Autodesk Fusion 360 part; units mm, degrees
sketch "Sketch1" plane through (0, 0, 0) normal (0, 0, 1) x (1, 0, 0)
  circle A0 centre (0, 0) radius 15
  dimension "d1" = 30
extrude "Extrude1" add sketch "Sketch1" along normal blind 6
sketch "Sketch2" plane through (0, 0, 6) normal (0, 0, 1) x (-1, 0, 0)
  circle A0 centre (0, 0) radius 15
  circle A1 centre (-2, -7) radius 12.5
  circle A2 centre (-11, -14) radius 7.5
  dimension "d4" = 25
  dimension "d5" = 15
  dimension "d6" = 7
  dimension "d7" = 2
  dimension "d8" = 14
  dimension "d9" = 11
extrude "Extrude2" add sketch "Sketch2" against normal blind 6 contours A0 A1 A2 picked at (-2.4117, -16.9728)
pattern_circular "C-Pattern1" count 3 over 360 about axis through (0, 0, 6) along (0, 0, 1) of "Extrude2"
sketch "Sketch3" plane through (0, 0, 6) normal (0, 0, 1) x (-1, 0, 0)
  arc A0 (9.6768, -11.4612) -> (14.3884, 4.2397) centre (0, 0) ccw
  arc A1 (19.1866, 4.8092) -> (14.3884, 4.2397) centre (17.6244, -2.5263) ccw
  arc A2 (19.1866, 4.8092) -> (5.0873, 14.111) centre (7.0622, 1.7679) ccw
  arc A3 (5.0873, 14.111) -> (-10.8659, 10.3408) centre (0, 0) ccw
  arc A4 (-13.7582, 14.2114) -> (-10.8659, 10.3408) centre (-6.6244, 16.5263) ccw
  arc A5 (-13.7582, 14.2114) -> (-14.7641, -2.6497) centre (-5.0622, 5.2321) ccw
  arc A6 (-14.7641, -2.6497) -> (-3.5225, -14.5805) centre (0, 0) ccw
  arc A7 (-5.4284, -19.0207) -> (-3.5225, -14.5805) centre (-11, -14) ccw
  arc A8 (-5.4284, -19.0207) -> (9.6768, -11.4612) centre (-2, -7) ccw
  circle A9 centre (0, 0) radius 12
  dimension "d14" = 24
extrude "Extrude3" cut sketch "Sketch3" against normal blind 2 draft -45 contours A9
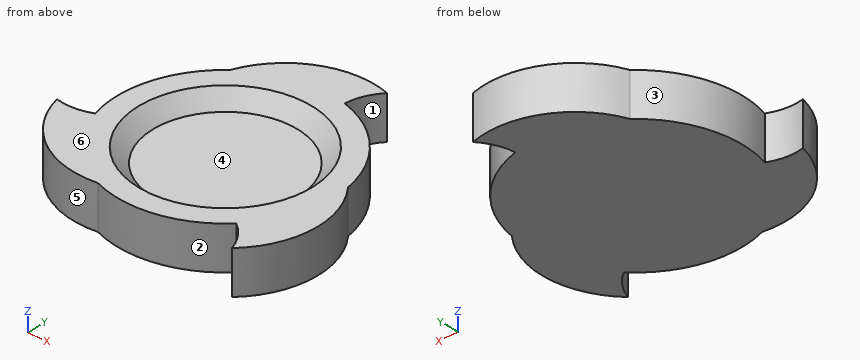
For this review, take the finished solid that the model builds, in its own axes (mm). Face numbers are marked on the shaded views. A direction names the side the tool comes from. Round coordinates to 2 decimals unless told otherwise and drop trailing zeros. Order: outer loops, then holes, each group sorted by start corner. A loop starts at its lowest first (then second) coordinate and runs counter-clockwise, first axis right, second up. Notation, with made-up numbers: (85.5, -38.5) -> (102.5, -38.5) arc R24 cw to (102.5, -19.5) -> close; hole circle Ø10 at (9, 79). An arc over 180 degrees is marked (long way). Put each result on its own line as item: value.
Q1. Add section B-B on x = 0. Write out the cut boundary in (y, z).
Check result:
outline: (-15, 0) -> (19.34, 0) -> (19.34, 6) -> (12, 6) -> (10, 4) -> (-10, 4) -> (-12, 6) -> (-15, 6) -> close
Q2. Add section C-C on y = 0. Write out the cut boundary in (x, z), plus the area to 3 significant figures.
Check result:
outline: (-15, 0) -> (16.41, 0) -> (16.41, 6) -> (12, 6) -> (10, 4) -> (-10, 4) -> (-12, 6) -> (-15, 6) -> close
area: 144 mm2
Q3. Add section D-D on x = -13.5. Write out the cut boundary in (y, z), plus the area to 3 significant figures.
Check result:
outline: (-12.48, 0) -> (6.54, 0) -> (6.54, 6) -> (-12.48, 6) -> close
area: 114 mm2
Q4. Insertion check: pin 1 Ø8 at (x, y) = (3, 8.5) entering from +Z; pin 2 Ø3 at (y, z) = (12.5, 5.5) entering from -X; pin 3 Ø2 at (x, z) = (-9.5, 4) entering from +Y; pin 4 Ø1.5 at (x, y) = (2, 4) entering from +Z. Each pin has a flat end and moves straight along its axis. Give the tip position at first contact, or say it passes through.
Check result:
pin 1: z = 6
pin 2: x = -10.2
pin 3: y = 13.78
pin 4: z = 4
Q5. For probe 1 along Z at (x, y) = (2.5, -3); probe 2 along Y at (x, z) = (-1, 5.25); probe 3 along X at (y, z) = (-13, 2.65), list the stretches that pass through material, from the lowest coordinate up. Write a range as [from, to].
Check result:
probe 1: [0, 4]
probe 2: [-14.97, -11.21], [11.21, 19.13]
probe 3: [-12.55, 7.48], [13.24, 14.86]
Q6. Mouldability with a two-part tool opening along Y and no side actions: class the marked faces 3, 4, 5 and 6 as pulls with the +Y half, pulls with the -Y half, needs draft (parallel to the pull), parting line crosses it, or undercut.
Check result:
face 3: undercut
face 4: undercut
face 5: pulls with the -Y half
face 6: needs draft
Q7. Add section A-A on z = 4.5. Write out the cut boundary in (x, y), plus the area to 3 significant figures.
Check result:
outline: (-19.19, -4.81) arc R12.5 ccw to (-5.09, -14.11) arc R15 ccw to (10.87, -10.34) arc R7.5 cw to (13.76, -14.21) arc R12.5 ccw to (14.76, 2.65) arc R15 ccw to (3.52, 14.58) arc R7.5 cw to (5.43, 19.02) arc R12.5 ccw to (-9.68, 11.46) arc R15 ccw to (-14.39, -4.24) arc R7.5 cw to start; hole circle Ø21 at (0, 0)
area: 505 mm2
Q8. Machinability: for the marked faces 1 and 2, which of the approach directions +Z, -Z, +X, -X, +Y, -Y give a long, thin tool a straight path to every point of the face, cutting with its end or side? Answer none if there is none.
Check result:
face 1: +Z, -Z, +X
face 2: +Z, -Z, -Y
